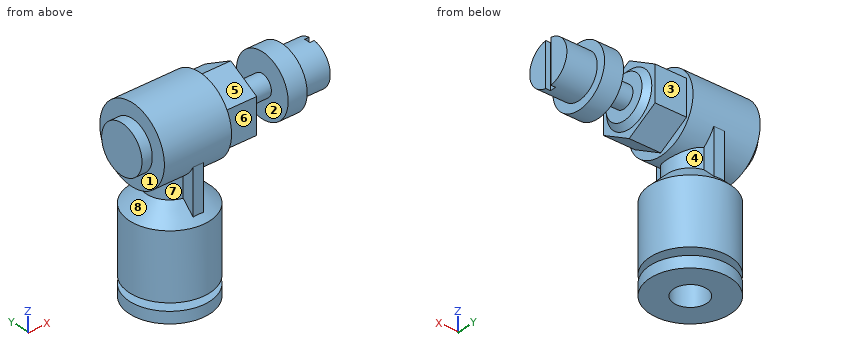
from build123d import *

# Parameters (mm, degrees)
SKETCH2_OUTSIDE_W   = 17.744
SKETCH2_OUTSIDE_H   = 17.744
CUT_EXTRUDE1_DEPTH  = 4.15
SKETCH3_W           = 6.384434702
SKETCH3_H           = 0.8
CUT_EXTRUDE2_DEPTH  = 0.6
SKETCH5_W           = 1.4
SKETCH5_H           = 8.9
BOSS_EXTRUDE1_DEPTH = 10


with BuildPart() as part:
    # Sketch1 → Revolve1 (revolve)
    with BuildSketch(Plane.XY):
        Polygon((0, 0), (0, 3.125), (1.35, 3.125), (1.35, 5), (14.35, 5), (14.35, 3.5), (15.05, 2.8), (15.05, 1.4), (18.5, 1.4), (18.5, 4), (21, 4), (21, 2.875), (25, 2.875), (25, 0), align=None)
    revolve(axis=Axis((25, 0, 0), (-1, 0, 0)))

    # Sketch2 outside → Cut-Extrude1 (cut)
    with BuildSketch(Plane(origin=(14.35, 0, 0), x_dir=(0, 0, -1), z_dir=(1, 0, 0))):
        Rectangle(SKETCH2_OUTSIDE_W, SKETCH2_OUTSIDE_H)
        Polygon((4.618802154, 0), (2.309401077, 4), (-2.309401077, 4), (-4.618802154, 0), (-2.309401077, -4), (2.309401077, -4), align=None, mode=Mode.SUBTRACT)
    extrude(amount=-CUT_EXTRUDE1_DEPTH, mode=Mode.SUBTRACT)

    # Sketch3 → Cut-Extrude2 (cut)
    with BuildSketch(Plane(origin=(25, 0, 0), x_dir=(0, 0, -1), z_dir=(1, 0, 0))):
        Rectangle(SKETCH3_W, SKETCH3_H)
    extrude(amount=-CUT_EXTRUDE2_DEPTH, mode=Mode.SUBTRACT)

    # Sketch4 → Revolve2 (revolve)
    with BuildSketch(Plane(origin=(0, 0, 0), x_dir=(1, 0, 0), z_dir=(0, 1, 0))):
        Polygon((6.3, 0), (6.3, 10.947554121), (4.15, 10.947554121), (4.15, 20), (1.05, 20), (1.05, 18.5), (3.7, 18.5), (3.7, 17.5), (1.05, 17.5), (1.05, 8.95), (3.3, 6.7), (3.3, 0), align=None)
    revolve(axis=Axis((6.3, 0, 0), (0, 0, -1)))

    # Sketch5 → Boss-Extrude1 (add)
    with BuildSketch(Plane.XY):
        with Locations((6.3, 0)):
            Rectangle(SKETCH5_W, SKETCH5_H)
    extrude(amount=-BOSS_EXTRUDE1_DEPTH)


solid = part.part
Design review of the part built by this model. Coordinates are the model's own, in mm. Face numbers are marked on the shaded views. A direction names the side the tool comes from. Round coordinates to 2 decimals unless told otherwise and drop trailing zeros. Loops run counter-clockwise (first coordinate to the right, second up) from the corner with the lowest first, then second, coordinate; pieces in that order, holes last. Notation, with made-up numbers: (5.5, 72) - (40.5, 72) arc R14 ccw to (40.5, 78) - close; hole circle Ø3 at (2, -16). An arc over 180 degrees is marked (long way). One line per question, with ' | ' between items.
1. We need section A-A, the plane x = 6.3. State the section outline as (y, z) points.
Results are:
outline: (-5.25, -20) - (-2.15, -20) - (-2.15, -10.95) - (2.15, -10.95) - (2.15, -20) - (5.25, -20) - (5.25, -18.5) - (2.6, -18.5) - (2.6, -17.5) - (5.25, -17.5) - (5.25, -8.95) - (4.45, -8.15) - (4.45, -2.28) arc R5 ccw (long way) to (-4.45, -2.28) - (-4.45, -8.15) - (-5.25, -8.95) - (-5.25, -17.5) - (-2.6, -17.5) - (-2.6, -18.5) - (-5.25, -18.5) - close
2. For the marked faces 4, 5, 6, 7 and 8, list the 3-axis set-ups (+Z, -Z, +X, -X, +Y, -Y) from which the entire face can be reached by the end or side of a thin tool; tool diameter is ignored.
Results are:
face 4: +X | face 5: +Z, +X, -Y | face 6: +Z, -Z, +X, -Y | face 7: -X | face 8: none
3. Clearance check with flat-ended pins moving along their axes: P1, Ø5, axis at y = 3, z = -1.5, coming from the +X side; P2, Ø1.3, axis at x = 6, y = 0.5, coming from the -Z side; P3, Ø1, axis at x = 12, y = 1, coming from the -Z side; P4, Ø1.5, axis at y = 2.5, z = -7, coming from the +X side. State where each tip first meets the part, or that it passes through.
Results are:
P1: stops at x = 25 | P2: stops at z = -10.95 | P3: stops at z = -4.33 | P4: stops at x = 9.63
4. We need section C-C, the plane x = 13. State the section outline as (y, z) points, and give its area (3 significant figures).
Results are:
outline: (-4, -2.31) - (0, -4.62) - (4, -2.31) - (4, 2.31) - (0, 4.62) - (-4, 2.31) - close | area: 55.4 mm²
5. For L1, parallel to Z at x = 10, y = 1.5; L2, parallel to Y at x = 6.3, z = -18; L3, parallel to Y at x = 6.3, z = -17, list the stretches that pass through material, from the lowest coordinate up. Write a range as [from, to].
Results are:
L1: z = [-20, -18.5], [-17.5, -7.69], [-4.77, 4.77] | L2: y = [-2.6, -2.15], [2.15, 2.6] | L3: y = [-5.25, -2.15], [2.15, 5.25]
6. Draft analysis for pull direction X (two halves, no side actions). For the marked faces 1, 2 and 3, state which applies: released by +X, released by -X, zero draft, split by the parting line, or undercut.
Results are:
face 1: released by -X | face 2: undercut | face 3: zero draft
7. We need section B-B, the plane z = -5.5. State the section outline as (x, y) points.
Results are:
outline: (5.6, -4.45) - (7, -4.45) - (7, -2.92) arc R3 ccw to (7, 2.92) - (7, 4.45) - (5.6, 4.45) - (5.6, 2.92) arc R3 ccw to (5.6, -2.92) - close
